Here's how the part is built. I have some questions about the finished solid (model axes, mm). Face numbers are marked on the shaded views. A direction names the side the tool comes from. Coordinates: 2 decimals unless noted, no trailing zeros. Write each loop counter-clockwise with the first axis right and the second up, starting at its lowest first coordinate (ties: lowest second). Pieces come first, ordered by that corner, then holes. Notation, with made-up numbers: M 17.25,-33.5 L 22.25,-33.5 A16 cw 22.25,-18.5 Z; hole C 9,24 d10. An arc over 180 degrees is marked long. Use a Markdown table: item, result.
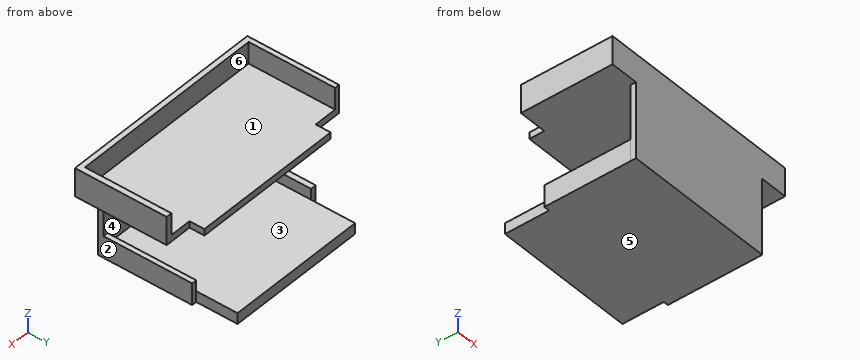
```python
from build123d import *

# Parameters (mm, degrees)
SKETCH_1_W      = 65
SKETCH_1_H      = 60
EXTRUDE_2_DEPTH = 5
SKETCH_2_W      = 2.242579202
SKETCH_2_H      = 40.913257232
EXTRUDE_3_DEPTH = 10
EXTRUDE_4_DEPTH = 10
SKETCH_4_W      = 69.848233062
SKETCH_4_H      = 2.620198038
EXTRUDE_6_DEPTH = 35
EXTRUDE_7_DEPTH = 3
EXTRUDE_9_DEPTH = 10


with BuildPart() as part:
    # 草图1 → 凸台-拉伸2 (new body)
    with BuildSketch(Plane.XY):
        with Locations((13.426561916, 13.374518887)):
            Rectangle(SKETCH_1_W, SKETCH_1_H)
    extrude(amount=EXTRUDE_2_DEPTH)

    # 草图2 → 凸台-拉伸3 (add)
    with BuildSketch(Plane(origin=(0, 0, 0), x_dir=(-1, 0, 0), z_dir=(0, 0, -1))):
        with Locations((-47.047851517, 3.831147503)):
            Rectangle(SKETCH_2_W, SKETCH_2_H)
    extrude(amount=-EXTRUDE_3_DEPTH)

    # 草图3 → 凸台-拉伸4 (add)
    with BuildSketch(Plane(origin=(0, 0, 0), x_dir=(-1, 0, 0), z_dir=(0, 0, -1))):
        Polygon((19.073438084, 23.061567441), (21.666178099, 23.061567441), (21.666178099, -16.667593717), (19.073438084, -16.625481113), align=None)
    extrude(amount=-EXTRUDE_4_DEPTH)

    # 草图4 → 凸台-拉伸6 (add)
    with BuildSketch(Plane(origin=(0, 0, 0), x_dir=(-1, 0, 0), z_dir=(0, 0, -1))):
        with Locations((-13.245024587, -17.935580132)):
            Rectangle(SKETCH_4_W, SKETCH_4_H)
    extrude(amount=-EXTRUDE_6_DEPTH)

    # 草图5 → 凸台-拉伸7 (add)
    with BuildSketch(Plane.XY.offset(35)):
        Polygon((-21.666178099, 23.061567441), (-34.613761508, 23.061567441), (-34.613761508, -19.245679151), (-21.679091944, -19.245679151), (48.169141118, -19.245679151), (60.804068806, -19.245679151), (60.804068806, 23.061567441), (48.169141118, 23.061567441), (48.169141118, 29.937605797), (-21.679091944, 29.937605797), align=None)
    extrude(amount=EXTRUDE_7_DEPTH)

    # 草图7 → 凸台-拉伸9 (add)
    with BuildSketch(Plane.XY.offset(38)):
        Polygon((-32.387714445, 23.061567441), (-34.613761508, 23.061567441), (-34.613761508, -19.245679151), (60.804068806, -19.245679151), (60.804068806, 23.061567441), (58.173614472, 23.061567441), (58.173614472, -16.803323091), (-32.387714445, -16.803323091), align=None)
    extrude(amount=EXTRUDE_9_DEPTH)


solid = part.part
```
1. Which directions (+Z, -Z, +X, -X, +Y, -Y) give clear straight access to the entire face, cutting with the end or side of a thin tool? Please do the marked faces 1, 2 and 3.
Answers follow:
| item | result |
|---|---|
| face 1 | +Z, +Y |
| face 2 | -Z, +X, +Y, -Y |
| face 3 | +Y |
2. Will these pins go through, and if not, where does the flat tip stop? pin 1 Ø0.9 at (y, z) = (27, 36.5) entering from +X; pin 2 Ø5 at (y, z) = (11, 5.5) entering from -X; pin 3 Ø11 at (x, z) = (34, 42) entering from +Y; pin 4 Ø10.5 at (y, z) = (-7, 17) entering from +X.
Answers follow:
| item | result |
|---|---|
| pin 1 | stops at x = 48.17 |
| pin 2 | stops at x = -21.67 |
| pin 3 | stops at y = 29.94 |
| pin 4 | passes through |
3. I need wall thicknesses on probe 1 along Z at (x, y) = (30.5, 6); probe 2 along Y at (x, z) = (37.5, 14); probe 3 along Z at (x, y) = (-20, 28.5). Which ranges of each line are inside material? Lowest first, please.
Answers follow:
| item | result |
|---|---|
| probe 1 | z = 0 to 5, 35 to 38 |
| probe 2 | y = -19.25 to -16.63 |
| probe 3 | z = 35 to 38 |
4. Suppose I cut it at C-C on x = 25.5. Write out the boundary of the cut face in (y, z), and give its area (3 significant figures).
Answers follow:
| item | result |
|---|---|
| outline | M -19.25,0 L 43.37,0 L 43.37,5 L -16.63,5 L -16.63,35 L 29.94,35 L 29.94,38 L -16.8,38 L -16.8,48 L -19.25,48 Z |
| area | 564 mm2 |
5. Suppose I cut it at A-A on y = -5. Write out the boundary of the cut face in (x, z).
Answers follow:
| item | result |
|---|---|
| outline | M -34.61,35 L 60.8,35 L 60.8,48 L 58.17,48 L 58.17,38 L -32.39,38 L -32.39,48 L -34.61,48 Z; M -21.67,0 L 48.17,0 L 48.17,10 L 45.93,10 L 45.93,5 L -19.07,5 L -19.07,10 L -21.67,10 Z |
6. Suppose I cut it at D-D on y = 38.5. Write out the boundary of the cut face in (x, z).
Answers follow:
| item | result |
|---|---|
| outline | M -19.07,0 L 45.93,0 L 45.93,5 L -19.07,5 Z |
7. We'd pull the mould along Z, two halves only. Please class the marked faces 4, 5 and 6: +Z half, -Z half, draft (parallel to the pull), parting line (faces both ways), or undercut.
Answers follow:
| item | result |
|---|---|
| face 4 | undercut |
| face 5 | -Z half |
| face 6 | draft |
